Source: three-view drawing plus pictorial views. Frame: mm from the lowest corner of the part. A direction names the side the tool comes from. Coordinates: 2 decimals unless noted, no trailing zeros. Order: outer loops, then holes, each group sorted by start corner. A loop starts at its lowest first (then second) coordinate and runs counter-clockwise, first axis right, second up. Notation, with made-up numbers: (-37, 57.5) - (-23, 57.5) arc R27 cw to (-23, 88.5) - close; hole circle Ø2 at (42, 68.5). An arc over 180 degrees is marked (long way). One line per question, with ' | ' between items.
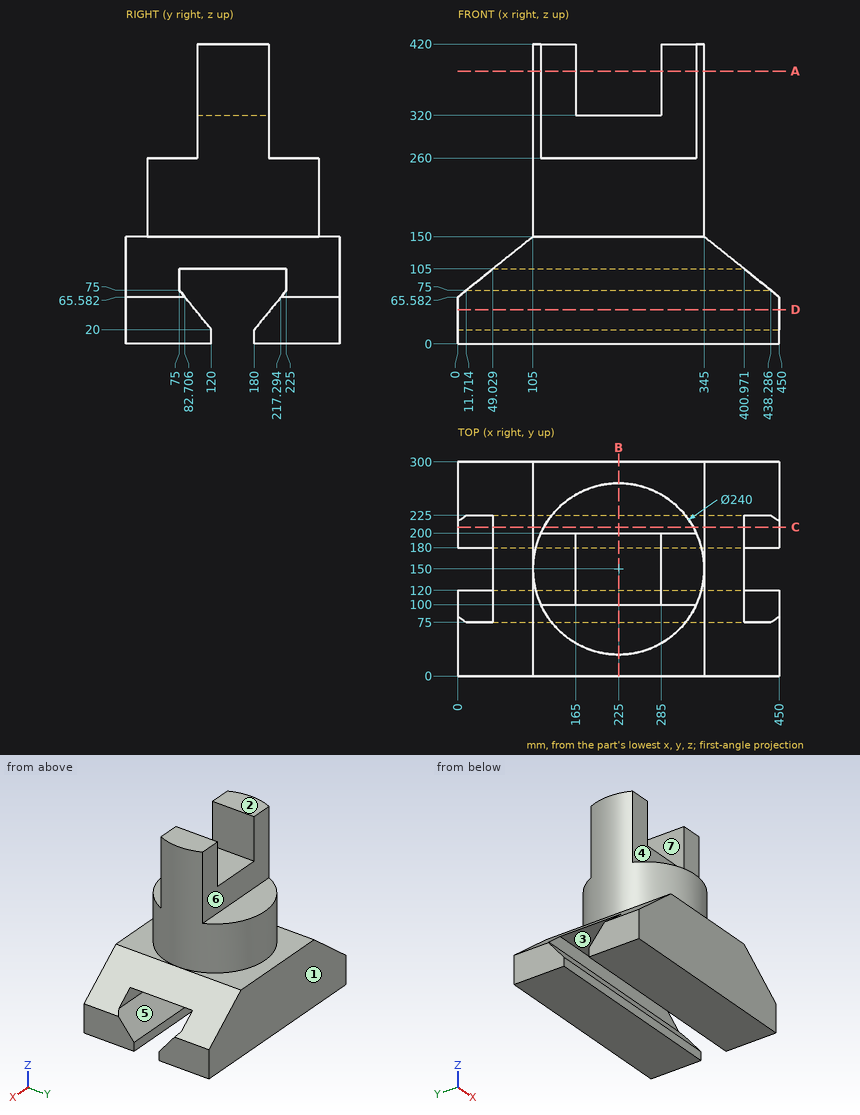
Item 1: Contact query for flat-ended pins moving along their axis: P1, Ø8, axis at y = 206, z = 293.5, coming from the +X side; P2, Ø12, axis at x = 291, z = 266.5, coming from the -Y side; P3, Ø10, axis at x = 382, y = 225, coming from the +Z side; P4, Ø1, axis at y = 181.5, z = 106, coming from the +X side. Output: stop coordinate, or through.
Data:
P1: through | P2: y = 100 | P3: z = 124.27 | P4: x = 400.35
Item 2: Section D-D on z = 48. Return the cut outline in (x, y), and give its area (3 significant figures).
Data:
outline: (0, 0) - (450, 0) - (450, 97.09) - (0, 97.09) - close; (0, 202.91) - (450, 202.91) - (450, 300) - (0, 300) - close | area: 87,400 mm^2
Item 3: Draft query along Y for the marked faces 1, 2 and 3. Return one class per face: released by +Y, released by -Y, zero draft, split by the parting line, or undercut.
Data:
face 1: released by +Y | face 2: zero draft | face 3: undercut
Item 4: Section B-B on x = 225. Return the cut outline in (y, z).
Data:
outline: (0, 0) - (120, 0) - (120, 20) - (75, 75) - (75, 105) - (225, 105) - (225, 75) - (180, 20) - (180, 0) - (300, 0) - (300, 150) - (270, 150) - (270, 260) - (200, 260) - (200, 320) - (100, 320) - (100, 260) - (30, 260) - (30, 150) - (0, 150) - close
Item 5: Ray query, line 1 (Y direction, x = 356.5, z = 76.5); line 2 (Z direction, x = 132.5, y = 55.5); line 3 (Y direction, x = 302.5, z = 282.5). Return the intervals inside material, ascending.
Data:
line 1: 0 to 75, 225 to 300 | line 2: 0 to 150 | line 3: 100 to 200
Item 6: Section C-C on y = 208.5. Return the cut outline in (x, z) (1 decimal), and give its area (3 significant figures).
Data:
outline: (0, 0) - (450, 0) - (450, 54.8) - (0, 54.8) - close; (49, 105) - (401, 105) - (345, 150) - (329.8, 150) - (329.8, 260) - (120.2, 260) - (120.2, 150) - (105, 150) - close | area: 61,000 mm^2
Item 7: Access query for the marked faces 4, 5, 6 and 7. Directions: +Z, -Z, +X, -X, +Y, -Y. A direction counts if a zero-diameter tool reaches every point of the face in a straight line with its end or side. Return the directions, or none.
Data:
face 4: +Z, +X, -X, -Y | face 5: +X, -X | face 6: +Z, +X, -X, +Y | face 7: +Z, +Y, -Y
Item 8: Section A-A on z = 382. Return the cut outline in (x, y), and give its area (3 significant figures).
Data:
outline: (115.91, 100) - (165, 100) - (165, 200) - (115.91, 200) arc R120 ccw to start; (285, 100) - (334.09, 100) arc R120 ccw to (334.09, 200) - (285, 200) - close | area: 11,300 mm^2
